```python
from build123d import *

# Parameters (mm, degrees)
F1_DEPTH = 100
F2_R     = 15
F3_W     = 25
F3_H     = 10
F4_DEPTH = 80
F5_R     = 4.99999
F6_R     = 10
F7_R     = 5


# Not quite as in the source:
# - a fillet or chamfer is up to 0.001 mm smaller than in the source, because OpenCascade refuses the exact size


with BuildPart() as f1:
    # F0 (on Right) → F1 (new body)
    with BuildSketch(Plane.YZ):
        Polygon((65, 0), (0, 0), (0, -30), (45, -30), align=None)
    extrude(amount=F1_DEPTH)

    # F2
    f2_edges = [f1.edges().sort_by_distance(p)[0] for p in [
        (50, 65, 0),
        (50, 0, -30),
    ]]
    fillet(f2_edges, radius=F2_R)

    # F3 (on face) → F4 (cut)
    with BuildSketch(Plane.YZ.offset(100)):
        with Locations((22.5, -15)):
            Rectangle(F3_W, F3_H)
    extrude(amount=-F4_DEPTH, mode=Mode.SUBTRACT)

    # F5 (radius 5 in the source; OpenCascade refuses exactly that, so slightly less here)
    f5_edges = [f1.edges().sort_by_distance(p)[0] for p in [
        (60, 10, -10),
        (60, 10, -20),
        (60, 35, -10),
        (60, 35, -20),
    ]]
    fillet(f5_edges, radius=F5_R)

    # F6
    f6_edges = [f1.edges().sort_by_distance(p)[0] for p in [
        (50, 0, 0),
        (50, 45, -30),
    ]]
    fillet(f6_edges, radius=F6_R)

    # F7
    f7_edges = [f1.edges().sort_by_distance(p)[0] for p in [
        (0, 23.486122, 0),
    ]]
    fillet(f7_edges, radius=F7_R)


solid = f1.part
```
Read the model definition and answer for the solid it produces. Units are mm, in the model's axes. A direction names the side the tool comes from. Give positions to 0.01 mm unless a question says otherwise; leave off trailing zeros. Order: outer loops, then holes, each group sorted by start corner. A loop starts at its lowest first (then second) coordinate and runs counter-clockwise, first axis right, second up. Notation, with made-up numbers: (17.25, 75.5) -> (58.25, 75.5) arc R19 cw to (58.25, 102.5) -> close; hole circle Ø11 at (-1, 59.5). An arc over 180 degrees is marked (long way). Write item = value, one per line.
1. Straight lines are drawn through the part: line 1 along Z through (x, y) = (40.5, 19.5); line 2 along X through (y, z) = (33, -16.5); line 3 along Z through (x, y) = (55.5, 14). For each, find the intervals that lie inside material, in ascending order.
Numbers:
line_1 = -30 to -20, -10 to 0
line_2 = 0 to 20
line_3 = -29.97 to -19.9, -10.1 to 0
2. Given pin 1 (2 mm diameter, centred on x = 19.5, z = -6, fed in from +Y); pin 2 (6 mm diameter, centred on x = 13.5, z = -23, fed in from +Y); pin 3 (1 mm diameter, centred on x = 44.5, z = -26.5, fed in from +Y), each flat-ended and moving along its own axis, determine where each tip first touches the part or whether it passes through.
Numbers:
pin_1 = 49.66
pin_2 = 51.11
pin_3 = 47.65
3. A cutting plane is placed at D-D, the plane y = 31.5. Write down the section's boundary in (x, z).
Numbers:
outline = (0, -25) arc R5 ccw to (5, -30) -> (100, -30) -> (100, -19.77) -> (20, -19.77) -> (20, -10.23) -> (100, -10.23) -> (100, 0) -> (5, 0) arc R5 ccw to (0, -5) -> close
4. A cutting plane is placed at C-C, the plane x = 18. Write down the section's boundary in (y, z), and give its area (3 significant figures).
Numbers:
outline = (0, -15) arc R15 ccw to (15, -30) -> (39.65, -30) arc R10 ccw to (47.97, -25.55) -> (49.45, -23.32) arc R15 ccw to (36.97, 0) -> (10, 0) arc R10 ccw to (0, -10) -> close
area = 1,400 mm²
5. A cutting plane is placed at B-B, the plane y = 24.5. Write down the section's boundary in (x, z).
Numbers:
outline = (0, -25) arc R5 ccw to (5, -30) -> (100, -30) -> (100, -20) -> (20, -20) -> (20, -10) -> (100, -10) -> (100, 0) -> (5, 0) arc R5 ccw to (0, -5) -> close
6. The mould has two halves that part along Y. Classify faces 3 (the face through (52, 0, -12)), 4 (the face through (53.2, 44.4, -28.8)), 5 (the face through (61, 22, -20)), 6 (the face through (52, 24, 0)): +Y half, -Y half, draft (parallel to the pull), parting line (faces both ways), or undercut.
Numbers:
face_3 = -Y half
face_4 = +Y half
face_5 = undercut
face_6 = draft
7. For faces 1 (the face through (59, 34, -12)), 2 (the face through (52, 27, -30)), determine the directions among +Z, -Z, +X, -X, +Y, -Y from which every point of the face is accessible in a straight line to the end or side of a thin tool.
Numbers:
face_1 = +X
face_2 = -Z, +X, -X, +Y, -Y
